Here's how the part is built. I have some questions about the finished solid (model axes, mm). Face numbers are marked on the shaded views. A direction names the side the tool comes from. Round coordinates to 2 decimals unless told otherwise and drop trailing zeros. Loops run counter-clockwise (first coordinate to the right, second up) from the corner with the lowest first, then second, coordinate; pieces in that order, holes last. Notation, with made-up numbers: (-1.75, -34.75) -> (31.25, -34.75) arc R22 ccw to (31.25, -21.75) -> close; hole circle Ø2 at (74, -39). An arc over 180 degrees is marked (long way). One line per item, written item: value. Start each with the question number.
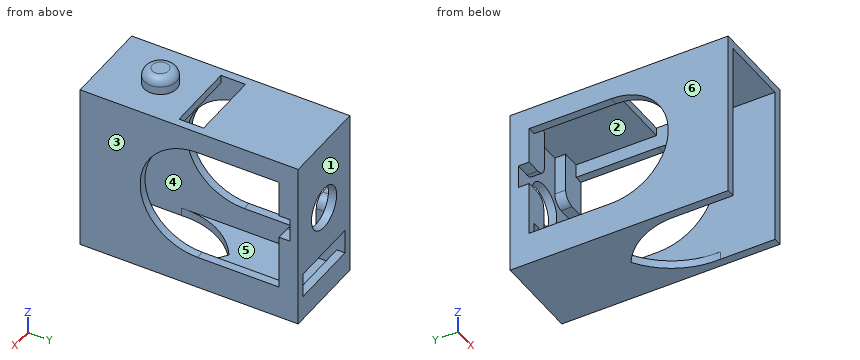
```python
from build123d import *

# Parameters (mm, degrees)
SKETCH1_W           = 16
SKETCH1_H           = 31
BOSS_EXTRUDE1_DEPTH = 40
SHELL1_T            = -1.5
SKETCH2_W           = 13
SKETCH2_H           = 4.5
CUT_EXTRUDE1_DEPTH  = 1.5
CUT_EXTRUDE2_DEPTH  = 1.5
SKETCH4_R           = 3.9
CUT_EXTRUDE3_DEPTH  = 1.5
SKETCH6_W           = 3
SKETCH6_H           = 7
BOSS_EXTRUDE2_DEPTH = 2
SKETCH7_W           = 3.2
SKETCH7_H           = 9.2
BOSS_EXTRUDE3_DEPTH = 2
SKETCH9_W           = 13
SKETCH9_H           = 4.5
CUT_EXTRUDE5_DEPTH  = 1.5
FILLET1_R           = 2
SKETCH10_R          = 3
BOSS_EXTRUDE4_DEPTH = 3
FILLET2_R           = 1.5
CUT_EXTRUDE6_DEPTH  = 55.881690936
SKETCH12_W          = 4.3
SKETCH12_H          = 2
CUT_EXTRUDE7_DEPTH  = 55.881690936


with BuildPart() as part:
    # Sketch1 → Boss-Extrude1 (new body)
    with BuildSketch(Plane(origin=(0, 0, 0), x_dir=(1, 0, 0), z_dir=(0, 1, 0))):
        with Locations((8, -15.5)):
            Rectangle(SKETCH1_W, SKETCH1_H)
    extrude(amount=BOSS_EXTRUDE1_DEPTH)

    # Shell1
    shell1_openings = [part.faces().sort_by_distance(p)[0] for p in [
        (8, 0, 15.5),
    ]]
    offset(amount=SHELL1_T, openings=shell1_openings, kind=Kind.INTERSECTION)

    # Sketch2 → Cut-Extrude1 (cut)
    with BuildSketch(Plane(origin=(0, 40, 0), x_dir=(1, 0, 0), z_dir=(0, 1, 0))):
        with Locations((8, -6.75)):
            Rectangle(SKETCH2_W, SKETCH2_H)
    extrude(amount=-CUT_EXTRUDE1_DEPTH, mode=Mode.SUBTRACT)

    # Sketch3 → Cut-Extrude2 (cut)
    with BuildSketch(Plane(origin=(0, 0, 0), x_dir=(-1, 0, 0), z_dir=(0, 0, -1))):
        with BuildLine():
            Line((-14.5, 10), (-14.5, -1))
            Line((-14.5, -1), (-1.5, -1))
            Line((-1.5, -1), (-1.5, 10))
            ThreePointArc((-1.5, 10), (-3.046805874, 17.164215382), (-8, 22.566479573))
            ThreePointArc((-8, 22.566479573), (-12.953194126, 17.164215382), (-14.5, 10))
        make_face()
    extrude(amount=-CUT_EXTRUDE2_DEPTH, mode=Mode.SUBTRACT)

    # Sketch4 → Cut-Extrude3 (cut)
    with BuildSketch(Plane(origin=(0, 40, 0), x_dir=(1, 0, 0), z_dir=(0, 1, 0))):
        with Locations(Location((8, -17.9, 0), (0, 0, 270))):
            Circle(SKETCH4_R)
    extrude(amount=-CUT_EXTRUDE3_DEPTH, mode=Mode.SUBTRACT)

    # Sketch6 → Boss-Extrude2 (add)
    with BuildSketch(Plane(origin=(0, 38.5, 0), x_dir=(-1, 0, 0), z_dir=(0, -1, 0))):
        with Locations((-13, -12.5)):
            Rectangle(SKETCH6_W, SKETCH6_H)
        with Locations((-3, -12.5)):
            Rectangle(SKETCH6_W, SKETCH6_H)
    extrude(amount=BOSS_EXTRUDE2_DEPTH)

    # Sketch7 → Boss-Extrude3 (add)
    with BuildSketch(Plane(origin=(0, 38.5, 0), x_dir=(-1, 0, 0), z_dir=(0, -1, 0))):
        with Locations((-12.9, -24.9)):
            Rectangle(SKETCH7_W, SKETCH7_H)
        with Locations((-3.1, -24.9)):
            Rectangle(SKETCH7_W, SKETCH7_H)
    extrude(amount=BOSS_EXTRUDE3_DEPTH)

    # Sketch9 → Cut-Extrude5 (cut)
    with BuildSketch(Plane.XY.offset(31)):
        with Locations((8, 19.497097074)):
            Rectangle(SKETCH9_W, SKETCH9_H)
    extrude(amount=-CUT_EXTRUDE5_DEPTH, mode=Mode.SUBTRACT)

    # Fillet1
    fillet1_edges = [part.edges().sort_by_distance(p)[0] for p in [
        (11.3, 37.5, 20.3),
        (4.7, 37.5, 20.3),
        (11.5, 37.5, 16),
        (4.5, 37.5, 16),
    ]]
    fillet(fillet1_edges, radius=FILLET1_R)

    # Sketch10 → Boss-Extrude4 (add)
    with BuildSketch(Plane.XY.offset(31)):
        with Locations((8, 10)):
            Circle(SKETCH10_R)
    extrude(amount=BOSS_EXTRUDE4_DEPTH)

    # Fillet2
    fillet2_edges = [part.edges().sort_by_distance(p)[0] for p in [
        (5, 10, 34),
    ]]
    fillet(fillet2_edges, radius=FILLET2_R)

    # Sketch11 → Cut-Extrude6 (cut, through all)
    with BuildSketch(Plane.ZY):
        with BuildLine():
            Line((6, 36.5), (27, 36.5))
            Line((27, 36.5), (27, 21.5))
            ThreePointArc((27, 21.5), (16.5, 11), (6, 21.5))
            Line((6, 21.5), (6, 36.5))
        make_face()
    extrude(amount=-CUT_EXTRUDE6_DEPTH, mode=Mode.SUBTRACT)

    # Sketch12 → Cut-Extrude7 (cut, through all)
    with BuildSketch(Plane(origin=(16, 0, 0), x_dir=(0, 0, -1), z_dir=(1, 0, 0))):
        with Locations((-18.15, 37.5)):
            Rectangle(SKETCH12_W, SKETCH12_H)
    extrude(amount=-CUT_EXTRUDE7_DEPTH, mode=Mode.SUBTRACT)


solid = part.part
```
Q1. I want a section at D-D on y = 5. Please give me the cut outline in (x, z), plus the area to 4 significant figures.
Q2. I want a section at C-C on z = 17.9. Please give me the cut outline in (x, y).
Q3. Which directions (+Z, -Z, +X, -X, +Y, -Y) give clear straight access to the entire face, cutting with the end or side of a thin tool? Please do the marked faces 5 and 6.
Q4. I want a section at B-B on x = 14. Please give me the cut outline in (y, z).
Q5. If we mould it in two halves opening along X, with no side actions, what happens to the marked faces 1, 2, 3 and 4? For each: released by +X, released by -X, zero draft, split by the parting line, or undercut.
Q6. Will these pins go through, and if not, where does the flat tip stop? P1, Ø1, axis at x = 5.5, z = 20.5, coming from the -Y side; P2, Ø2, axis at x = 15, y = 37.5, coming from the +Z side; P3, Ø8, axis at x = 5, y = 4.5, coming from the +Z side.
Q7. If I drill on line 1 along X through (y, z) = (2.5, 7); line 2 along Z through (x, y) = (4.25, 31); line 3 along X through (y, z) = (39.2, 17.9), over which ranges is the centre line in solid material (lowest first)?
Q8. I want a section at A-A on y = 25.5. Please give me the cut outline in (x, z).
Answers below:
1. outline: (0, 0) -> (1.5, 0) -> (1.5, 29.5) -> (14.5, 29.5) -> (14.5, 0) -> (16, 0) -> (16, 31) -> (0, 31) -> close
1. area: 112.5 mm^2
2. outline: (0, 0) -> (1.5, 0) -> (1.5, 11.09) -> (0, 11.09) -> close; (0, 38.5) -> (4.1, 38.5) -> (4.1, 40) -> (0, 40) -> close; (11.9, 38.5) -> (16, 38.5) -> (16, 40) -> (11.9, 40) -> close; (14.5, 0) -> (16, 0) -> (16, 11.09) -> (14.5, 11.09) -> close
3. face 5: -Y
3. face 6: +Z, -Z, -X, +Y, -Y
4. outline: (0, 29.5) -> (17.25, 29.5) -> (17.25, 31) -> (0, 31) -> close; (14.51, 0) -> (40, 0) -> (40, 4.5) -> (38.5, 4.5) -> (38.5, 1.5) -> (14.51, 1.5) -> close; (21.75, 29.5) -> (36.5, 29.5) -> (36.5, 20.3) -> (38.5, 20.3) -> (38.5, 16) -> (36.5, 16) -> (36.5, 9) -> (40, 9) -> (40, 31) -> (21.75, 31) -> close
5. face 1: zero draft
5. face 2: undercut
5. face 3: released by +X
5. face 4: undercut
6. P1: stops at y = 38.5
6. P2: stops at z = 31
6. P3: stops at z = 33.79
7. line 1: x = 0 to 1.5, 14.5 to 16
7. line 2: z = 0 to 1.5, 29.5 to 31
7. line 3: x = 0 to 4.1, 11.9 to 16
8. outline: (0, 0) -> (16, 0) -> (16, 6) -> (14.5, 6) -> (14.5, 1.5) -> (1.5, 1.5) -> (1.5, 6) -> (0, 6) -> close; (0, 27) -> (1.5, 27) -> (1.5, 29.5) -> (14.5, 29.5) -> (14.5, 27) -> (16, 27) -> (16, 31) -> (0, 31) -> close
